The drawing under review shows one solid part. Ordinate dimensions are in mm from its lowest x, y, z. A direction names the side the tool comes from. Coordinates: 2 decimals unless noted, no trailing zeros. Order: outer loops, then holes, each group sorted by start corner. A loop starts at its lowest first (then second) coordinate and runs counter-clockwise, first axis right, second up.
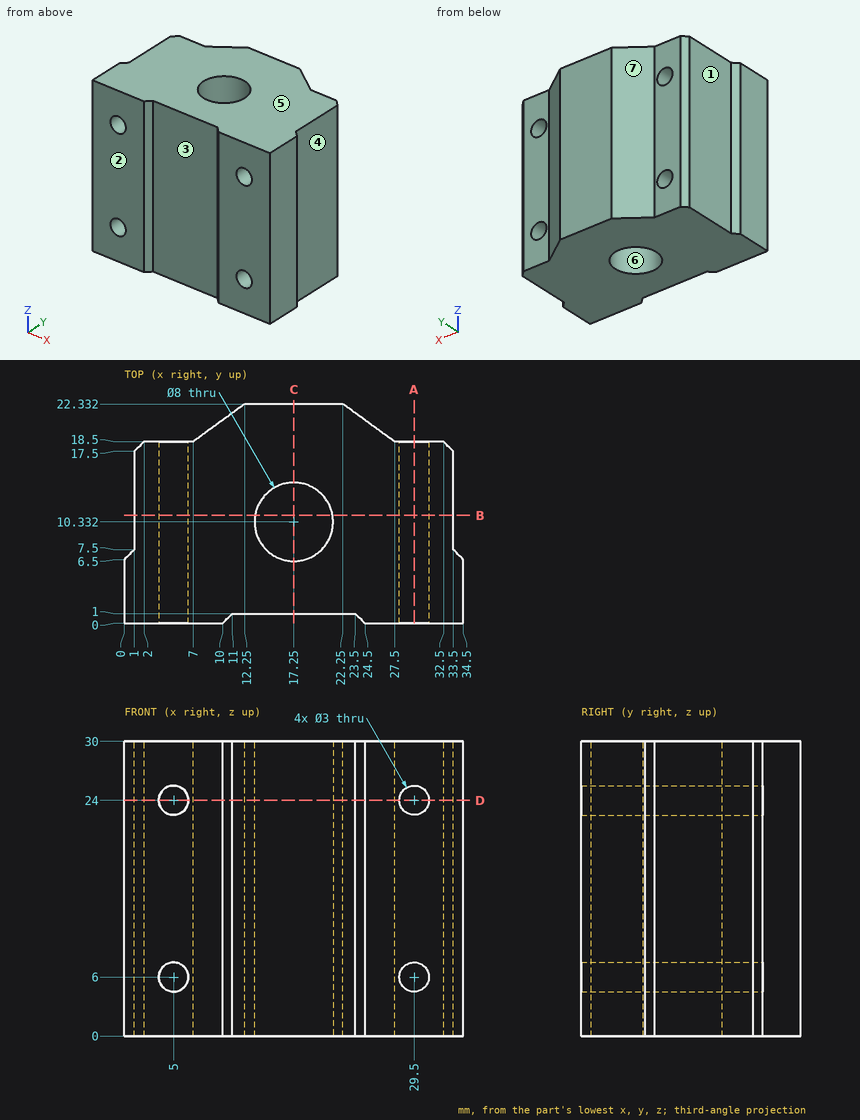
(1) Draft analysis for pull direction Y (two halves, no side actions). For the marked faces 5, 6 and 7, state which applies: released by +Y, released by -Y, zero draft, split by the parting line, or undercut.
A:
face 5: zero draft
face 6: undercut
face 7: released by +Y
(2) Machinability: for the marked faces 1, 2, 3 and 4, which of the approach directions +Z, -Z, +X, -X, +Y, -Y give a long, thin tool a straight path to every point of the face, cutting with its end or side? Answer none if there is none.
A:
face 1: +Z, -Z, -X, +Y
face 2: +Z, -Z, +X, -X, -Y
face 3: +Z, -Z, -Y
face 4: +Z, -Z, +X, +Y
(3) We need section A-A, the plane x = 29.5. Write out the cut boundary in (y, z), and give its area (3 significant figures).
A:
outline: (0, 0) - (18.5, 0) - (18.5, 4.5) - (0, 4.5) - close; (0, 7.5) - (18.5, 7.5) - (18.5, 22.5) - (0, 22.5) - close; (0, 25.5) - (18.5, 25.5) - (18.5, 30) - (0, 30) - close
area: 444 mm2
(4) For pin 1 Ø1.5 at (x, z) = (6.5, 23) entering from +Y; pin 2 Ø5 at (x, z) = (28.5, 18.5) entering from +Y (1 decimal); pin 3 Ø4 at (x, z) = (30, 10) entering from +Y, all flat-tipped, find the tip position at first contact; note any pin that passes through.
A:
pin 1: stops at y = 18.68
pin 2: stops at y = 19.6
pin 3: stops at y = 18.5
(5) Wall thickness on probe 1 along X at (y, z) = (10.5, 6); probe 2 along Z at (x, y) = (5, 13.75); probe 3 along Z at (x, y) = (30.5, 16.25): over which ranges is each line inside the solid? List them lowest first.
A:
probe 1: x = 1 to 3.5, 6.5 to 13.25, 21.25 to 28, 31 to 33.5
probe 2: z = 0 to 4.5, 7.5 to 22.5, 25.5 to 30
probe 3: z = 0 to 4.88, 7.12 to 22.88, 25.12 to 30
(6) We need section C-C, the plane x = 17.25. Write out the cut boundary in (y, z), and give its area (3 significant figures).
A:
outline: (1, 0) - (6.33, 0) - (6.33, 30) - (1, 30) - close; (14.33, 0) - (22.33, 0) - (22.33, 30) - (14.33, 30) - close
area: 400 mm2
(7) We need section D-D, the plane z = 24. Write out the cut boundary in (x, y).
A:
outline: (0, 0) - (3.5, 0) - (3.5, 18.5) - (2, 18.5) - (1, 17.5) - (1, 7.5) - (0, 6.5) - close; (6.5, 0) - (10, 0) - (11, 1) - (23.5, 1) - (24.5, 0) - (28, 0) - (28, 18.5) - (27.5, 18.5) - (22.25, 22.33) - (12.25, 22.33) - (7, 18.5) - (6.5, 18.5) - close; (31, 0) - (34.5, 0) - (34.5, 6.5) - (33.5, 7.5) - (33.5, 17.5) - (32.5, 18.5) - (31, 18.5) - close; hole circle Ø8 at (17.25, 10.33)
(8) We need section B-B, the plane y = 11. Write out the cut boundary in (x, z), and give its area (3 significant figures).
A:
outline: (1, 0) - (13.31, 0) - (13.31, 30) - (1, 30) - close; (21.19, 0) - (33.5, 0) - (33.5, 30) - (21.19, 30) - close; hole circle Ø3 at (5, 6); hole circle Ø3 at (5, 24); hole circle Ø3 at (29.5, 6); hole circle Ø3 at (29.5, 24)
area: 710 mm2
